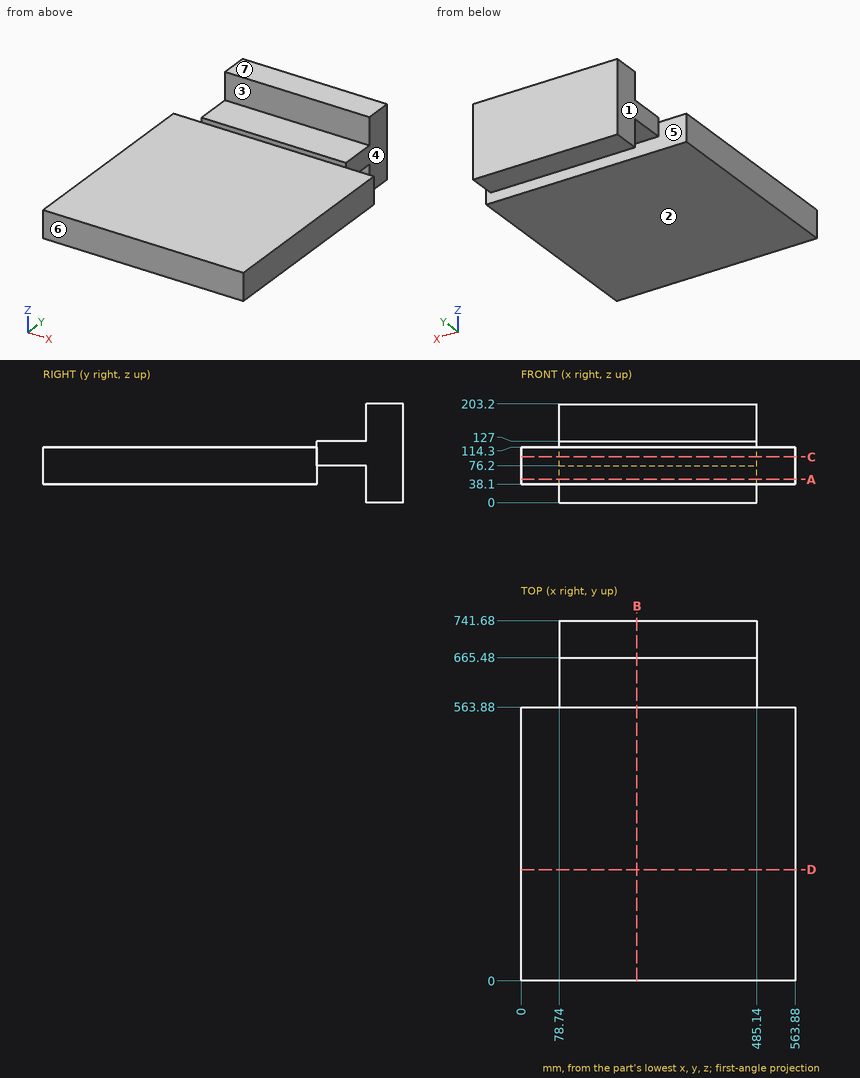
The figure shows three views and two pictorial views of one solid part (mm, origin at its lowest corner). Answer the questions. A direction names the side the tool comes from. Give positions to 0.01 mm unless a question says otherwise; leave off trailing zeros. Write each loop counter-clockwise with the first axis right and the second up, starting at its lowest first coordinate (ties: lowest second). Pieces come first, ordered by that corner, then holes. Notation, with made-up numbers: (70.5, 62.25) - (98.5, 62.25) arc R15 cw to (98.5, 86.25) - close; hole circle Ø6 at (62, 54.5). An arc over 180 degrees is marked (long way). Use one line per item in the form item = value.
1. Determine the mould class of the marked faces 5, 6 and 7 for opening direction Y: released by +Y, released by -Y, zero draft, split by the parting line, or undercut.
Filled in:
face_5 = undercut
face_6 = released by -Y
face_7 = zero draft
2. Consider L1, parallel to Z at x = 259, y = 175; L2, parallel to Y at x = 350.5, z = 71; L3, parallel to X at y = 671, z = 44. Determine where each line is inside the solid, lowest interval first.
Filled in:
L1 = 38.1 to 114.3
L2 = 0 to 563.88, 665.48 to 741.68
L3 = 78.74 to 485.14
3. A cutting plane is placed at A-A (z = 48). Write down the section's boundary in (x, y).
Filled in:
outline = (0, 0) - (563.88, 0) - (563.88, 563.88) - (0, 563.88) - close; (78.74, 665.48) - (485.14, 665.48) - (485.14, 741.68) - (78.74, 741.68) - close
4. A cutting plane is placed at C-C (z = 94.5). Write down the section's boundary in (x, y).
Filled in:
outline = (0, 0) - (563.88, 0) - (563.88, 563.88) - (485.14, 563.88) - (485.14, 741.68) - (78.74, 741.68) - (78.74, 563.88) - (0, 563.88) - close
5. Each of these flat-tipped pins is pushed along its axis until it touches: pin 1 Ø10 at (x, y) = (87.5, 542) entering from -Z; pin 2 Ø5 at (x, y) = (262.5, 607.5) entering from -Z; pin 3 Ø14 at (x, z) = (302, 123) entering from -Y. Where does it stop, or does it pass through?
Filled in:
pin_1 = 38.1
pin_2 = 76.2
pin_3 = 563.88
6. A cutting plane is placed at D-D (y = 229). Write down the section's boundary in (x, z).
Filled in:
outline = (0, 38.1) - (563.88, 38.1) - (563.88, 114.3) - (0, 114.3) - close
7. A cutting plane is placed at B-B (x = 238.5). Write down the section's boundary in (y, z).
Filled in:
outline = (0, 38.1) - (563.88, 38.1) - (563.88, 76.2) - (665.48, 76.2) - (665.48, 0) - (741.68, 0) - (741.68, 203.2) - (665.48, 203.2) - (665.48, 127) - (563.88, 127) - (563.88, 114.3) - (0, 114.3) - close
8. For the marked faces 1, 2, 3 and 4, determine the directions among +Z, -Z, +X, -X, +Y, -Y from which every point of the face is accessible in a straight line to the end or side of a thin tool.
Filled in:
face_1 = +Z, -Z, -X, +Y
face_2 = -Z, +X, -X, -Y
face_3 = +Z, +X, -X, -Y
face_4 = +Z, -Z, +X, +Y
